Work out the finished part from the listing and answer in its coordinate system (mm). A direction names the side the tool comes from. Round coordinates to 2 decimals unless told otherwise and drop trailing zeros. Order: outer loops, then holes, each group sorted by start corner. A loop starts at its lowest first (then second) coordinate and runs counter-clockwise, first axis right, second up. Notation, with made-up numbers: (-1, -18.5) - (36, -18.5) arc R19 cw to (36, 1.5) - close; hole circle Ø1 at (-22, 40.5). An arc over 180 degrees is marked (long way). One line per question, with ' | ' between items. Start each with the question number.
from build123d import *

# Parameters (mm, degrees)
SKETCH1_W           = 19
SKETCH1_H           = 9
BOSS_EXTRUDE1_DEPTH = 2
BOSS_EXTRUDE2_DEPTH = 2
SKETCH4_R           = 1.5
CUT_EXTRUDE1_DEPTH  = 2
SKETCH5_R           = 1.5
CUT_EXTRUDE2_DEPTH  = 2


with BuildPart() as part:
    # Sketch1 → Boss-Extrude1 (new body)
    with BuildSketch(Plane(origin=(0, 0, 0), x_dir=(1, 0, 0), z_dir=(0, 1, 0))):
        with Locations((9.5, 4.5)):
            Rectangle(SKETCH1_W, SKETCH1_H)
    extrude(amount=BOSS_EXTRUDE1_DEPTH)

    # Sketch3 → Boss-Extrude2 (add)
    with BuildSketch(Plane.XY):
        with BuildLine():
            Line((0, 2), (19, 2))
            ThreePointArc((19, 2), (9.5, 9), (0, 2))
        make_face()
    extrude(amount=-BOSS_EXTRUDE2_DEPTH)

    # Sketch4 → Cut-Extrude1 (cut)
    with BuildSketch(Plane(origin=(0, 2, 0), x_dir=(1, 0, 0), z_dir=(0, 1, 0))):
        with Locations((5, 5)):
            Circle(SKETCH4_R)
        with Locations((14, 5)):
            Circle(SKETCH4_R)
    extrude(amount=-CUT_EXTRUDE1_DEPTH, mode=Mode.SUBTRACT)

    # Sketch5 → Cut-Extrude2 (cut)
    with BuildSketch(Plane.XY):
        with Locations((9.5, 4.5)):
            Circle(SKETCH5_R)
    extrude(amount=-CUT_EXTRUDE2_DEPTH, mode=Mode.SUBTRACT)


solid = part.part
1) Section C-C on y = 4.5 is taken. Give the vertices of the cut face in (x, z), and give its area (3 significant figures).
2) Section B-B on z = -5 is taken. Give the vertices of the cut face in (x, y).
3) For faces 4 (the flat face through (9, 2, -6)), 5 (the flat face through (19, 1, -4)), determine the directions among +Z, -Z, +X, -X, +Y, -Y from which every point of the face is accessible in a straight line to the end or side of a thin tool.
4) Determine the mould class of faces 1 (the cylindrical face through (9.68, 9, -0.99)), 2 (the flat face through (9, 1, -9)), 3 (the cylindrical face through (12.5, 1.01, -5.07)) for opening direction X: released by +X, released by -X, zero draft, split by the parting line, or undercut.
5) Section D-D on y = 1.25 is taken. Give the vertices of the cut face in (x, z).
6) Straight lines are drawn through the part: line 1 (X direction, y = 1.4, z = -5); line 2 (Z direction, x = 5, y = 1.5); line 3 (Y direction, x = 7.25, z = -4.75). For each, find the intervals that lie inside material, in ascending order.
7) Section A-A on x = 9.5 is taken. Give the vertices of the cut face in (y, z), and give its area (3 significant figures).
8) Flat-ended cylindrical pins translate along their axes: pin 1 (3 mm diameter, centred on x = 7, y = 5, fed in from -Z); pin 2 (1.5 mm diameter, centred on y = 6, z = -2.5, fed in from -X). Find the tip coordinate at first contact, or state that the pin passes through.
Recorded:
1) outline: (1.18, -2) - (8, -2) - (8, 0) - (1.18, 0) - close; (11, -2) - (17.82, -2) - (17.82, 0) - (11, 0) - close | area: 27.3 mm²
2) outline: (0, 0) - (3.5, 0) - (3.5, 2) - (0, 2) - close; (6.5, 0) - (12.5, 0) - (12.5, 2) - (6.5, 2) - close; (15.5, 0) - (19, 0) - (19, 2) - (15.5, 2) - close
3) face 4: -Z, +X, -X, +Y | face 5: +Z, -Z, +X, +Y, -Y
4) face 1: split by the parting line | face 2: zero draft | face 3: undercut
5) outline: (0, -9) - (19, -9) - (19, 0) - (0, 0) - close; hole circle Ø3 at (5, -5); hole circle Ø3 at (14, -5)
6) line 1: x = 0 to 3.5, 6.5 to 12.5, 15.5 to 19 | line 2: z = -9 to -6.5, -3.5 to 0 | line 3: y = 0 to 2
7) outline: (0, -9) - (2, -9) - (2, -2) - (3, -2) - (3, 0) - (0, 0) - close; (6, -2) - (9, -2) - (9, 0) - (6, 0) - close | area: 26.0 mm²
8) pin 1: stops at z = -2 | pin 2: stops at x = 1.88
